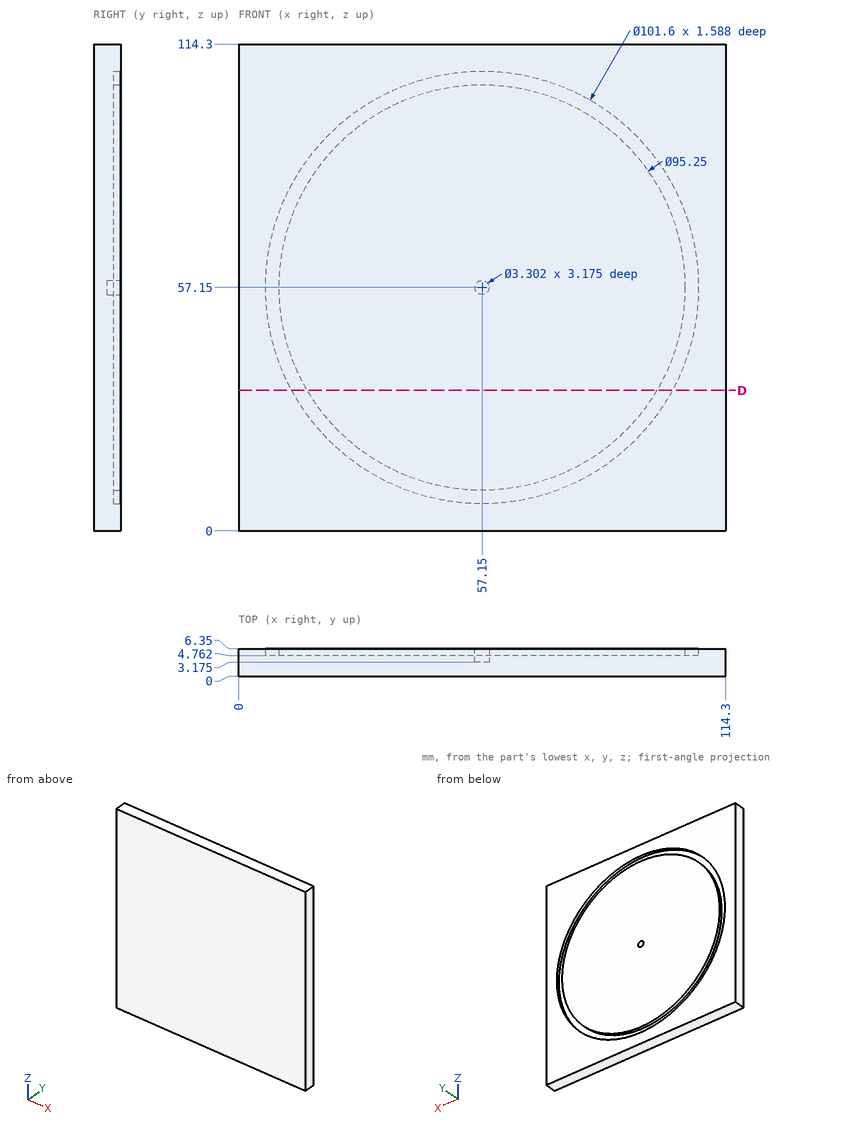
Job drawing, mm, ordinate dimensions from the low corner. One solid piece. Give positions to 0.01 mm unless a question says otherwise; leave off trailing zeros. Order: outer loops, then holes, each group sorted by start corner. A loop starts at its lowest first (then second) coordinate and runs counter-clockwise, first axis right, second up. Notation, with made-up numbers: (23.5, -37.75) -> (69.5, -37.75) arc R22 cw to (69.5, -18.75) -> close; hole circle Ø7 at (81, 20.5). An arc over 180 degrees is marked (long way). Return JSON: item names as keys, results as strings.
Q1. Flat gauge pin, fed straight in: pin 1 (1 mm diameter, centred on x = 57.5, z = 57, fed in from +Y) (1 decimal). Where does the tip first touch, or does it go through?
Working result:
{"pin 1": "y = 3.2"}
Q2. Drill centre lines: line 1 (Z direction, x = 88, y = 5) (1 decimal); line 2 (Z direction, x = 58, y = 6.25) (1 decimal); line 3 (X direction, y = 5.5, z = 61) (1 decimal). Where is each one in solid material? Low to high.
Working result:
{"line 1": "0 to 16.8, 20.9 to 93.4, 97.5 to 114.3", "line 2": "0 to 6.4, 9.5 to 55.7, 58.6 to 104.8, 107.9 to 114.3", "line 3": "0 to 6.5, 9.7 to 104.6, 107.8 to 114.3"}
Q3. Saw through at D-D (z = 33). Write the cut outline in (x, y).
Working result:
{"outline": "(0, 0) -> (114.3, 0) -> (114.3, 6.35) -> (101.84, 6.35) -> (101.84, 4.76) -> (98.2, 4.76) -> (98.2, 6.35) -> (16.1, 6.35) -> (16.1, 4.76) -> (12.46, 4.76) -> (12.46, 6.35) -> (0, 6.35) -> close"}
